Can you work these out from the model? Positions are in its coordinate system, mm. Round coordinates to 2 decimals unless told otherwise and drop trailing zeros. Loops run counter-clockwise (first coordinate to the right, second up) from the corner with the lowest first, then second, coordinate; pieces in that order, holes last.
(1) If I drill on line 1 along Y through (x, z) = (43.5, -49); line 2 along Y through (x, z) = (23, -33.5); line 3 along Z through (x, y) = (42.5, 279), over which ranges is the centre line in solid material (lowest first)?
(2) I want a section at B-B on z = -25.5. Write out the boundary of the cut face in (x, y).
(3) I want a section at A-A on x = 6.5. Write out the boundary of the cut face in (y, z), plus the area to 3 significant figures.
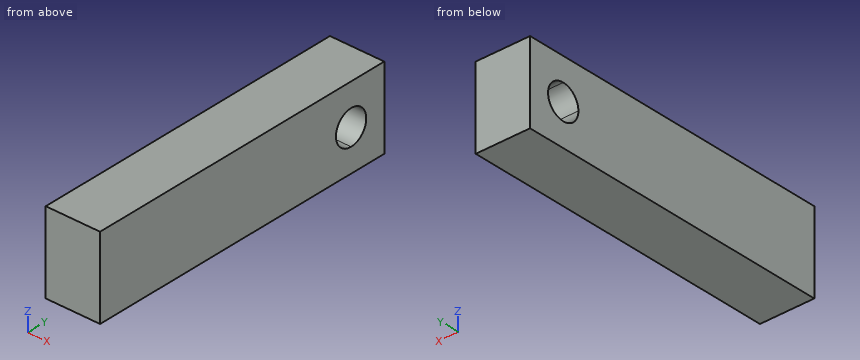
from build123d import *

# Parameters (mm, degrees)
SKETCH1_W           = 50.8
SKETCH1_H           = 76.2
BOSS_EXTRUDE1_DEPTH = 300
CUT_EXTRUDE1_DEPTH  = 150


with BuildPart() as part:
    # Sketch1 → Boss-Extrude1 (new body)
    with BuildSketch(Plane(origin=(0, 0, 0), x_dir=(1, 0, 0), z_dir=(0, 1, 0))):
        with Locations((25.4, 38.1)):
            Rectangle(SKETCH1_W, SKETCH1_H)
    extrude(amount=BOSS_EXTRUDE1_DEPTH)

    # Sketch2 → Cut-Extrude1 (cut)
    with BuildSketch(Plane(origin=(50.8, 0, 0), x_dir=(0, 0, -1), z_dir=(1, 0, 0))):
        with BuildLine():
            ThreePointArc((22, 265), (26.686291501, 253.686291501), (38, 249))
            Line((38, 249), (38, 265))
            Line((38, 265), (22, 265))
        make_face()
        with BuildLine():
            Line((38, 265), (38, 249))
            ThreePointArc((38, 249), (49.313708499, 253.686291501), (54, 265))
            ThreePointArc((54, 265), (38, 281), (22, 265))
            Line((22, 265), (38, 265))
        make_face()
    extrude(amount=-CUT_EXTRUDE1_DEPTH, mode=Mode.SUBTRACT)


solid = part.part
Filled sheet:
1. line 1: y = 0 to 253.38, 276.62 to 300
1. line 2: y = 0 to 249.65, 280.35 to 300
1. line 3: z = -76.2 to -45.75, -30.25 to 0
2. outline: (0, 0) - (50.8, 0) - (50.8, 255.01) - (0, 255.01) - close; (0, 274.99) - (50.8, 274.99) - (50.8, 300) - (0, 300) - close
3. outline: (0, -76.2) - (300, -76.2) - (300, 0) - (0, 0) - close; hole circle Ø32 at (265, -38)
3. area: 22,100 mm2
